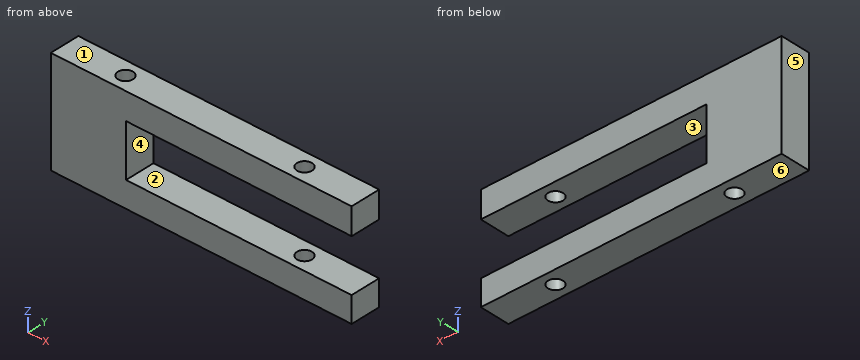
from build123d import *

# Parameters (mm, degrees)
BOSS_EXTRUDE1_DEPTH = 100
CUT_EXTRUDE1_REACH  = 619.562
SKETCH8_R           = 25


with BuildPart() as part:
    # Sketch5 → Boss-Extrude1 (new body)
    with BuildSketch(Plane(origin=(0, 0, 0), x_dir=(-1, 0, 0), z_dir=(0, -1, 0))):
        Polygon((-500, 171.192494481), (500, 171.192494481), (500, -177.207505519), (-500, -177.207505519), (-500, -88.603752759), (250, -88.603752759), (250, 85.596247241), (-500, 85.596247241), align=None)
    extrude(amount=BOSS_EXTRUDE1_DEPTH)

    # Cut-Extrude1: up to this face of the body (flat: up to its plane)
    cut_extrude1_end = Plane(part.part.faces().sort_by_distance((0, -50, 177.207505519))[0])
    # Sketch8 → Cut-Extrude1 (cut, up to the picked face)
    with BuildSketch(Plane(origin=(0, 0, -171.192494481), x_dir=(-1, 0, 0), z_dir=(0, 0, -1)), mode=Mode.PRIVATE) as cut_extrude1_sk1:
        with Locations((-297.6, -50)):
            Circle(SKETCH8_R)
    cut_extrude1_tool1 = split(extrude(cut_extrude1_sk1.sketch, amount=-CUT_EXTRUDE1_REACH, mode=Mode.PRIVATE), bisect_by=cut_extrude1_end, keep=Keep.BOTH, mode=Mode.PRIVATE)
    # Sketch8 → Cut-Extrude1 (cut, up to the picked face)
    with BuildSketch(Plane(origin=(0, 0, -171.192494481), x_dir=(-1, 0, 0), z_dir=(0, 0, -1)), mode=Mode.PRIVATE) as cut_extrude1_sk2:
        with Locations((297.6, -50)):
            Circle(SKETCH8_R)
    cut_extrude1_tool2 = split(extrude(cut_extrude1_sk2.sketch, amount=-CUT_EXTRUDE1_REACH, mode=Mode.PRIVATE), bisect_by=cut_extrude1_end, keep=Keep.BOTH, mode=Mode.PRIVATE)
    add(cut_extrude1_tool1.solids().sort_by(Axis((297.6, -50, -171.192494), (0, 0, 1)))[0], mode=Mode.SUBTRACT)
    add(cut_extrude1_tool2.solids().sort_by(Axis((-297.6, -50, -171.192494), (0, 0, 1)))[0], mode=Mode.SUBTRACT)


solid = part.part
Geometry: final body of the model. Coordinates: model frame, mm. Face numbers are marked on the shaded views. A direction names the side the tool comes from. Give positions to 0.01 mm unless a question says otherwise; leave off trailing zeros. Write each loop counter-clockwise with the first axis right and the second up, starting at its lowest first coordinate (ties: lowest second). Pieces come first, ordered by that corner, then holes. Notation, with made-up numbers: (49, 25) - (101, 25) arc R20 cw to (101, 59) - close; hole circle Ø3 at (41.25, 14.25). An arc over 180 degrees is marked (long way). Return JSON: item names as keys, results as strings. Group by question number.
1) Line query: line 1 (Z direction, x = 412, y = -82); line 2 (Y direction, x = 297.6, z = 134); line 3 (X direction, y = -51, z = 135). Output: solid intervals per line, ascending.
2) Section B-B on x = -297.6. Return the cut outline in (y, z).
3) First-contact query: P1, Ø4, axis at y = -68.5, z = -38.5, coming from the +X side. Flat tip, straight axial feed; report the tip coordinate or a pass-through.
4) Section D-D on x = 297.6. Return the cut outline in (y, z).
5) Section A-A on y = -50. Return the cut outline in (x, z).
6) Mould query, pull axis Z, two halves, no side actions, for the marked faces 3, 4, 5 and 6. Classes: released by +Z, released by -Z, zero draft, split by the parting line, or undercut.
7) Section C-C on z = 61.5. Return the cut outline in (x, y), plus the area to 3 significant figures.
8) Set-up query: the marked faces 1 and 2. Return all of +Z, -Z, +X, -X, +Y, -Y with unobstructed straight access to the full face (end or side cutting, diameter ignored); none if empty.
Filled in:
{
 "1": {"line 1": "z = -171.19 to -85.6, 88.6 to 177.21", "line 2": "y = -100 to -75, -25 to 0", "line 3": "x = -500 to -322.58, -272.62 to 272.62, 322.58 to 500"},
 "2": {"outline": "(-100, -171.19) - (-75, -171.19) - (-75, 177.21) - (-100, 177.21) - close; (-25, -171.19) - (0, -171.19) - (0, 177.21) - (-25, 177.21) - close"},
 "3": {"P1": "stops at x = -250"},
 "4": {"outline": "(-100, -171.19) - (-75, -171.19) - (-75, -85.6) - (-100, -85.6) - close; (-100, 88.6) - (-75, 88.6) - (-75, 177.21) - (-100, 177.21) - close; (-25, -171.19) - (0, -171.19) - (0, -85.6) - (-25, -85.6) - close; (-25, 88.6) - (0, 88.6) - (0, 177.21) - (-25, 177.21) - close"},
 "5": {"outline": "(-500, -171.19) - (-322.6, -171.19) - (-322.6, 177.21) - (-500, 177.21) - close; (-272.6, -171.19) - (272.6, -171.19) - (272.6, -85.6) - (-250, -85.6) - (-250, 88.6) - (272.6, 88.6) - (272.6, 177.21) - (-272.6, 177.21) - close; (322.6, -171.19) - (500, -171.19) - (500, -85.6) - (322.6, -85.6) - close; (322.6, 88.6) - (500, 88.6) - (500, 177.21) - (322.6, 177.21) - close"},
 "6": {"face 3": "undercut", "face 4": "undercut", "face 5": "zero draft", "face 6": "released by -Z"},
 "7": {"outline": "(-500, -100) - (-250, -100) - (-250, 0) - (-500, 0) - close; hole circle Ø50 at (-297.6, -50)", "area": "23,000 mm^2"},
 "8": {"face 1": "+Z, +X, -X, +Y, -Y", "face 2": "+X, +Y, -Y"}
}
